Build history of the part. All positions in model axes, mm. Round coordinates to 2 decimals unless told otherwise and drop trailing zeros. Return JSON: item names as keys, results as strings.
from build123d import *

# Parameters (mm, degrees)
SKETCH2_W           = 75
SKETCH2_H           = 5
BOSS_EXTRUDE1_DEPTH = 5
BOSS_EXTRUDE2_DEPTH = 5
LPATTERN1_COUNT     = 23
LPATTERN1_PITCH     = 3


with BuildPart() as part:
    # Sketch2 → Boss-Extrude1 (new body)
    with BuildSketch(Plane(origin=(0, 0, 0), x_dir=(1, 0, 0), z_dir=(0, 1, 0))):
        with Locations((4.747191011, 2.5)):
            Rectangle(SKETCH2_W, SKETCH2_H)
    extrude(amount=BOSS_EXTRUDE1_DEPTH)

    # Sketch2_3 → Boss-Extrude2 (add)
    with BuildSketch(Plane(origin=(0, 0, 0), x_dir=(1, 0, 0), z_dir=(0, 1, 0))):
        with BuildLine():
            ThreePointArc((-27.202808989, 7.25), (-27.639277587, 6.164470102), (-27.752808989, 5))
            Line((-27.752808989, 5), (-25.752808989, 5))
            ThreePointArc((-25.752808989, 5), (-25.86634039, 6.164470102), (-26.302808989, 7.25))
            Line((-26.302808989, 7.25), (-27.202808989, 7.25))
        make_face()
    boss_extrude2 = extrude(amount=BOSS_EXTRUDE2_DEPTH)

    # LPattern1: Boss-Extrude2 ×23
    with Locations(*[(i * LPATTERN1_PITCH, 0, 0) for i in range(1, LPATTERN1_COUNT)]):
        add(boss_extrude2)


solid = part.part
Q1. Pin check, flat tips, straight feed: pin 1 Ø1.1 at (x, y) = (-10, 2) entering from -Z; pin 2 Ø0.6 at (x, y) = (41, 3.5) entering from -Z. Stop position of each tip, or through.
Verdict:
{"pin 1": "stops at z = -6.75", "pin 2": "stops at z = -5"}
Q2. Wall check: L1, parallel to Z at x = -4.5, y = 0.85. Give the ranges that are in metal, low to high.
Verdict:
{"L1": "z = -5 to 0"}
Q3. Two-plate mould, pull along X, no slides. Class faces 1 (the cylindrical face through (-27.635, 2.465, -6.18)), 2 (the cylindrical face through (-13.862, 2.465, -6.148)): +X half, -X half, draft (parallel to the pull), parting line (faces both ways), or undercut.
Verdict:
{"face 1": "-X half", "face 2": "undercut"}
